Design review of the part built by this model. Coordinates are the model's own, in mm. A direction names the side the tool comes from. Round coordinates to 2 decimals unless told otherwise and drop trailing zeros. Write each loop counter-clockwise with the first axis right and the second up, starting at its lowest first coordinate (ties: lowest second). Pieces come first, ordered by that corner, then holes. Notation, with made-up numbers: (47.5, 11) - (57.5, 11) arc R35 ccw to (57.5, 44) - close; hole circle Ø4 at (12, 70). An arc over 180 degrees is marked (long way). Use one line per item in the form item = value.
Autodesk Inventor part; units mm, degrees
ref_plane "YZ Plane" through (0, 0, 0) normal (1, 0, 0) x (0, 1, 0)
ref_plane "XZ Plane" through (0, 0, 0) normal (0, 1, 0) x (-1, 0, 0)
ref_plane "XY Plane" through (0, 0, 0) normal (0, 0, 1) x (1, 0, 0)
sketch "Esboço1" plane through (0, 0, 0) normal (0, 0, 1) x (1, 0, 0)
  line L0 (-10, 7.5) -> (10, 7.5)
  line L1 (10, 7.5) -> (10, -7.5)
  line L2 (10, -7.5) -> (-10, -7.5)
  line L3 (-10, -7.5) -> (-10, 7.5)
  line L4 (-10, 7.5) -> (10, -7.5) construction
  line L5 (10, 7.5) -> (-10, -7.5) construction
  circle A0 centre (-1.5, 0) radius 1.5
  point P0 (0, 0)
  dimension "d0" = 20
  dimension "d1" = 15
  dimension "d13" = 3
  dimension "d14" = 1.5
  dimension "d15" = 7.5
extrude "Extrusão1" add sketch "Esboço1" against normal blind 3
sketch "Esboço2" plane through (0, 0, -3) normal (0, 0, -1) x (-1, 0, 0)
  line L0 (10, 7.5) -> (-10, 7.5)
  line L1 (-4, 7.5) -> (-4, -7.5247)
  line L2 (-7, 7.5) -> (-7, -7.5)
  line L3 (-10, -7.5) -> (10, -7.5)
  line L4 (-3, 7.5) -> (-3, -7.5247)
  line L5 (-8, 7.5) -> (-8, -7.5)
  point P0 (0, 0)
  point P1 (0, 0)
  point P2 (-3, -7.5)
  point P3 (-4, -7.5)
  dimension "d6" = 3
  dimension "d7" = 1
  dimension "d8" = 1
  dimension "d16" = 7
extrude "Extrusão2" add sketch "Esboço2" along normal blind 10 contours L4 L3 L1 L0 | L2 L3 L5 L0
sketch "Esboço3" plane through (-10, 7.5, 0) normal (0, 1, 0) x (1, 0, 0)
  point P0 (10, 0)
fillet "Arredondamento1" radius 5 1 edges at (10, 0, 0)
sketch "Esboço4" plane through (0, 0, -3) normal (0, 0, -1) x (-1, 0, 0)
  line L0 (-7, 7.5) -> (-7, -7.5)
  line L1 (-7, -7.5) -> (-4, -7.5)
  line L2 (-4, -7.5) -> (-4, 7.5)
  line L3 (-4, 7.5) -> (-7, 7.5)
  point P0 (0, 0)
extrude "Extrusão3" add sketch "Esboço4" along normal blind 7
fillet "Arredondamento3" radius 4 4 edges at (3.5, 7.5, -13) (7.5, 7.5, -13) (3.5, -7.5, -13) (7.5, -7.5, -13)
Q1. We need section D-D on z = -7.75. Write out the cut boundary in (x, y).
Calculated:
outline = (3, -7.5) - (8, -7.5) - (8, 7.5) - (3, 7.5) - close
Q2. For P1, Ø5, axis at y = 0, z = -1.5, coming from the +X side; P2, Ø0.9, axis at y = -2.5, z = -11, coming from the +X side; P3, Ø3.5, axis at y = 2.5, z = -11.5, coming from the -X side; P4, Ø4, axis at x = -0.5, y = 3, coming from the -Z side, all flat-tipped, find the tip position at first contact; note any pin that passes through.
Calculated:
P1 = 10
P2 = 8
P3 = 3
P4 = -3
Q3. We need section A-A on x = -1.5. Write out the cut boundary in (y, z), then the cut area to 3 significant figures.
Calculated:
outline = (-7.5, -3) - (-1.5, -3) - (-1.5, 0) - (-7.5, 0) - close; (1.5, -3) - (7.5, -3) - (7.5, 0) - (1.5, 0) - close
area = 36.0 mm2
Q4. Machinability: for faces 1 (the flat face through (7, 0, -11)), 2 (the flat face through (-4, 0, -3)), 3 (the flat face through (8, 0, -8)), which of the approach directions +Z, -Z, +X, -X, +Y, -Y give a long, thin tool a straight path to every point of the face, cutting with its end or side? Answer none if there is none.
Calculated:
face_1 = -Z, +Y, -Y
face_2 = -Z, -X, +Y, -Y
face_3 = -Z, +X, +Y, -Y
Q5. To check wall thickness, follow line 1 along Y through (x, z) = (-1.5, -0.8); line 2 along Z through (x, y) = (-4.75, -5.5); line 3 along X through (y, z) = (-5, -5). State the ranges of each line that lie inside material, in increasing order. Write a range as from..to.
Calculated:
line_1 = -7.5..-1.5, 1.5..7.5
line_2 = -3..0
line_3 = 3..8
Q6. We need section C-C on y = -2.25. Write out the cut boundary in (x, z).
Calculated:
outline = (-10, -3) - (3, -3) - (3, -13) - (4, -13) - (4, -10) - (7, -10) - (7, -13) - (8, -13) - (8, -3) - (10, -3) arc R5 ccw to (5.42, 0) - (-10, 0) - close
Q7. We need section B-B on y = 0. Write out the cut boundary in (x, z), then the cut area to 3 significant figures.
Calculated:
outline = (-10, -3) - (-3, -3) - (-3, 0) - (-10, 0) - close; (0, -3) - (3, -3) - (3, -13) - (4, -13) - (4, -10) - (7, -10) - (7, -13) - (8, -13) - (8, -3) - (10, -3) arc R5 ccw to (5.42, 0) - (0, 0) - close
area = 88.2 mm2
Q8. Draft analysis for pull direction X (two halves, no side actions). For faces 4 (the cylindrical face through (-2.7, -0.9, -1.5)), 5 (the flat face through (2, -7.5, -2)), 6 (the flat face through (3, 0, -8)), state which applies: released by +X, released by -X, zero draft, split by the parting line, or undercut.
Calculated:
face_4 = undercut
face_5 = zero draft
face_6 = released by -X
